Source: CAD feature listing. Evaluate the final solid. Frame: model axes, mm. A direction names the side the tool comes from. Give positions to 0.01 mm unless a question says otherwise; leave off trailing zeros. Loops run counter-clockwise (first coordinate to the right, second up) from the corner with the lowest first, then second, coordinate; pieces in that order, holes last. Notation, with made-up numbers: M 3,8.25 L 36,8.25 A9 ccw 36,25.25 Z; hole C -38,22 d7. An arc over 180 degrees is marked long. Answer in a Markdown table with one row per item.
```python
from build123d import *


with BuildPart() as f1:
    # F0 (on Front) → F1 (revolve)
    with BuildSketch(Plane.XZ):
        with BuildLine():
            Line((-26.9748, 0), (-9.525, 0))
            Line((-9.525, 0), (-9.525, 53.975))
            Line((-9.525, 53.975), (-26.9748, 53.975))
            Line((-26.9748, 53.975), (-26.9748, 44.830383))
            Line((-26.9748, 44.830383), (-25.517052, 44.830383))
            ThreePointArc((-25.517052, 44.830383), (-21.895214, 41.329264), (-25.408524, 37.719251))
            ThreePointArc((-25.408524, 37.719251), (-25.4508, 37.719), (-25.493076, 37.719251))
            Line((-25.493076, 37.719251), (-26.9748, 37.719251))
            Line((-26.9748, 37.719251), (-26.9748, 15.37081))
            Line((-26.9748, 15.37081), (-25.4508, 15.37081))
            ThreePointArc((-25.4508, 15.37081), (-22.77999, 12.7), (-25.4508, 10.02919))
            Line((-25.4508, 10.02919), (-26.9748, 10.02919))
            Line((-26.9748, 10.02919), (-26.9748, 0))
        make_face()
        with BuildLine():
            ThreePointArc((-25.493076, 37.719251), (-25.4508, 37.719), (-25.408524, 37.719251))
            Line((-25.408524, 37.719251), (-25.493076, 37.719251))
        make_face()
    revolve(axis=Axis((0, 0, 17.05089), (0, 0, 1)))


solid = f1.part
```
Q1. Reachability of faces 1 (the flat face through (-24, 10, 44.83)), 2 (the cylindrical face through (7.559, 5.796, 27.365)) from +Z, -Z, +X, -X, +Y, -Y: full face, straight path, thin tool, end or side. Return the list, or none.
Values follow:
| item | result |
|---|---|
| face 1 | none |
| face 2 | +Z, -Z |
Q2. Section query B-B (z = 7). Output: boundary loops of the cut face in (x, y) (3 decimals).
Values follow:
| item | result |
|---|---|
| outline | C 0,0 d53.95; hole C 0,0 d19.05 |
Q3. Section query D-D (z = 14). Output: boundary loops of the cut face in (x, y) (3 decimals).
Values follow:
| item | result |
|---|---|
| outline | C 0,0 d46.235; hole C 0,0 d19.05 |
Q4. Ray query, probe 1 along Z at (x, y) = (8, 24) (3 decimals); probe 2 along X at (y, z) = (0, 32) (3 decimals). Return the intervals inside material, ascending. Write a range as from..to.
Values follow:
| item | result |
|---|---|
| probe 1 | 0..10.034, 15.366..37.722, 44.828..53.975 |
| probe 2 | -26.975..-9.525, 9.525..26.975 |
Q5. Section query A-A (x = 0). Output: boundary loops of the cut face in (y, z) (3 decimals), plus the area to 3 significant figures.
Values follow:
| item | result |
|---|---|
| outline | M -26.975,0 L -9.525,0 L -9.525,53.975 L -26.975,53.975 L -26.975,44.83 L -25.517,44.83 A3.556 cw long -25.409,37.719 L -26.975,37.719 L -26.975,15.371 L -25.451,15.371 A2.671 cw -25.451,10.029 L -26.975,10.029 Z; M 9.525,0 L 26.975,0 L 26.975,10.029 L 25.451,10.029 A2.671 cw 25.451,15.371 L 26.975,15.371 L 26.975,37.719 L 25.409,37.719 A3.556 cw long 25.517,44.83 L 26.975,44.83 L 26.975,53.975 L 9.525,53.975 Z |
| area | 1,780 mm^2 |
Q6. Contact query for flat-ended pins moving along their axis: pin 1 Ø16 at (x, y) = (13, -5.5) entering from -Z; pin 2 Ø10 at (y, z) = (5.5, 5.5) entering from +X; pin 3 Ø6 at (y, z) = (15, 13) entering from -X; pin 4 Ø15 at (x, y) = (0, 0) entering from -Z. Output: stop coordinate, or through.
Values follow:
| item | result |
|---|---|
| pin 1 | z = 0 |
| pin 2 | x = 26.97 |
| pin 3 | x = -23.55 |
| pin 4 | through |
Q7. Mould query, pull axis Z, two halves, no side actions, for faces 3 (the cylindrical face through (5.848, 26.333, 49.339)), 4 (the flat face through (-20, -16, 15.371)), 5 (the flat face through (12, 0, 53.975)). Classes: +Z half, -Z half, draft (parallel to the pull), parting line (faces both ways), or undercut.
Values follow:
| item | result |
|---|---|
| face 3 | draft |
| face 4 | undercut |
| face 5 | +Z half |
